Input: part model. Units: mm. Frame: model coordinates. Round coordinates to 2 decimals unless told otherwise and drop trailing zeros. Loops run counter-clockwise (first coordinate to the right, second up) from the corner with the lowest first, then second, coordinate; pieces in that order, holes last. Notation, with made-up numbers: M 54.25,53.25 L 70.25,53.25 A8 cw 70.25,59.25 Z; hole C 22,-24.5 d3. An arc over 180 degrees is marked long. Put each result on its own line as item: value. Start each with the question number.
1) Pin query (flat end, axial travel): pin 1 (1.5 mm diameter, centred on y = -6, z = -7, fed in from -X); pin 2 (4 mm diameter, centred on y = -15, z = -7, fed in from +X). Return the tip coordinate at first contact, or that it passes through.
2) Section B-B on y = -3.5. Output: boundary loops of the cut face in (x, z) (3 decimals).
3) Line query: probe 1 along X at (y, z) = (6, 3.5); probe 2 along X at (y, z) = (-0.5, -8.25); probe 3 along Y at (x, z) = (153.5, 8.75). Output: solid intervals per line, ascending.
4) Section C-C on x = 155. Output: boundary loops of the cut face in (y, z) (3 decimals), plus the area to 3 significant figures.
from build123d import *

# Parameters (mm, degrees)
F0_W     = 38.1
F0_H     = 19.05
F1_DEPTH = 177.8
F4_DEPTH = 50.8
F6_DEPTH = 50.8


with BuildPart() as f1:
    # F0 (on Right) → F1 (new body, symmetric)
    with BuildSketch(Plane.YZ):
        Rectangle(F0_W, F0_H)
    extrude(amount=F1_DEPTH, both=True)

    # F3 (on face) → F4 (cut)
    with BuildSketch(Plane.XY.offset(9.525)):
        Polygon((-177.8, 19.05), (-177.8, -19.0363529205), (-139.7136470795, 19.05), align=None)
    extrude(amount=-F4_DEPTH, mode=Mode.SUBTRACT)

    # F5 (on face) → F6 (cut)
    with BuildSketch(Plane.XY.offset(9.525)):
        Polygon((138.9227120697, 19.05), (177.0227120697, -19.05), (177.8, -19.05), (177.8, 19.05), align=None)
    extrude(amount=-F6_DEPTH, mode=Mode.SUBTRACT)


solid = f1.part
Geometry results:
1. pin 1: stops at x = -165.51
1. pin 2: stops at x = 174.97
2. outline: M -162.264,-9.525 L 161.473,-9.525 L 161.473,9.525 L -162.264,9.525 Z
3. probe 1: x = -152.76 to 151.97
3. probe 2: x = -159.26 to 158.47
3. probe 3: y = -19.05 to 4.47
4. outline: M -19.05,-9.525 L 2.973,-9.525 L 2.973,9.525 L -19.05,9.525 Z
4. area: 420 mm²
